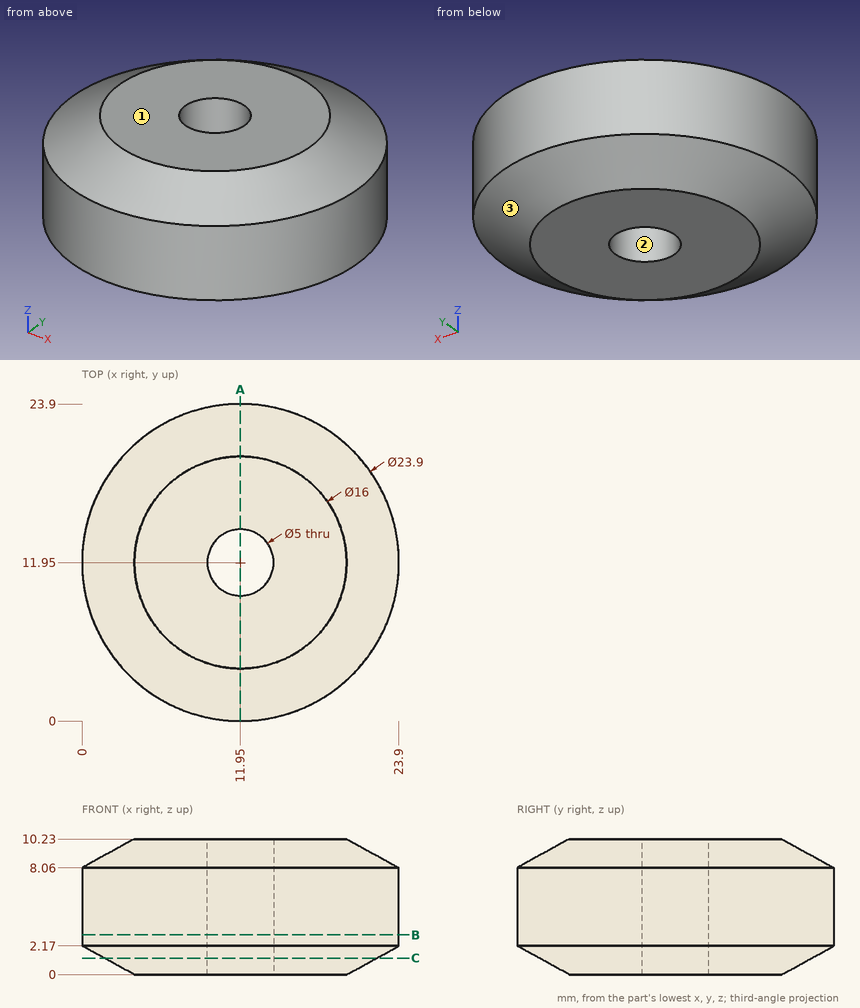
Study the drawing (mm; zero at the part's minimum x, y, z) and answer. Coordinates: 2 decimals unless noted, no trailing zeros. Loops run counter-clockwise (first coordinate to the right, second up) from the corner with the lowest first, then second, coordinate; pieces in that order, holes last. Notation, with made-up numbers: (71, -24.75) -> (86, -24.75) arc R19 ccw to (86, 1.25) -> close; hole circle Ø6 at (88.25, 20.25). An arc over 180 degrees is marked (long way). Answer in a Markdown table with one row per item. Add a question column.
1. Determine the mould class of the marked faces 1, 2 and 3 for opening direction X: +X half, -X half, draft (parallel to the pull), parting line (faces both ways), or undercut.
2. Flat-ended cylindrical pins translate along their axes: P1, Ø4, axis at x = 20, y = 11, coming from the -Z side; P2, Ø1.5, axis at y = 7.5, z = 4, coming from the -X side; P3, Ø2, axis at x = 5.5, z = 3, coming from the -Y side; P4, Ø6, axis at x = 7.5, z = 7, coming from the +Y side. Find the tip coordinate at first contact, or state that the pin passes through.
3. The part is cut by section C-C, the plane z = 1.25. Write down the section's boundary in (x, y), then the cut area to 3 significant figures.
4. Consider line 1 (Y direction, x = 11.95, z = 5.5); line 2 (X direction, y = 12.75, z = 8.5); line 3 (X direction, y = 10.5, z = 5.25). Determine where each line is inside the solid, lowest interval first. Write a range as [from, to].
5. The part is cut by section A-A, the plane x = 11.95. Write down the section's boundary in (y, z).
6. The part is cut by section B-B, the plane z = 3. Write down the section's boundary in (x, y), then the cut area to 3 significant figures.
Answer below:
| question | item | result |
|---|---|---|
| 1 | face 1 | draft |
| 1 | face 2 | undercut |
| 1 | face 3 | parting line |
| 2 | P1 | z = 0 |
| 2 | P2 | x = 0.59 |
| 2 | P3 | y = 1.32 |
| 2 | P4 | y = 23.81 |
| 3 | outline | circle Ø20.55 at (11.95, 11.95); hole circle Ø5 at (11.95, 11.95) |
| 3 | area | 312 mm2 |
| 4 | line 1 | [0, 9.45], [14.45, 23.9] |
| 4 | line 2 | [0.83, 9.58], [14.32, 23.07] |
| 4 | line 3 | [0.09, 9.91], [13.99, 23.81] |
| 5 | outline | (0, 2.17) -> (3.95, 0) -> (9.45, 0) -> (9.45, 10.23) -> (3.95, 10.23) -> (0, 8.06) -> close; (14.45, 0) -> (19.95, 0) -> (23.9, 2.17) -> (23.9, 8.06) -> (19.95, 10.23) -> (14.45, 10.23) -> close |
| 6 | outline | circle Ø23.9 at (11.95, 11.95); hole circle Ø5 at (11.95, 11.95) |
| 6 | area | 429 mm2 |
